Autodesk Inventor part; units mm, degrees
ref_plane "YZ Plane" through (0, 0, 0) normal (1, 0, 0) x (0, 1, 0)
ref_plane "XZ Plane" through (0, 0, 0) normal (0, 1, 0) x (-1, 0, 0)
ref_plane "XY Plane" through (0, 0, 0) normal (0, 0, 1) x (1, 0, 0)
sketch "Sketch1" plane through (0, 0, 0) normal (1, 0, 0) x (0, 1, 0)
  line L0 (1.27, -4.5) -> (-1.27, -4.5)
  line L1 (-1.27, -4.5) -> (-1.27, 4.5)
  line L2 (-1.27, 4.5) -> (1.27, 4.5)
  line L3 (1.27, 4.5) -> (1.27, -4.5)
  line L4 (1.27, -4.5) -> (-1.27, 4.5) construction
  line L5 (-1.27, -4.5) -> (1.27, 4.5) construction
  point P0 (0, 0)
  point P1 (0, 0)
  dimension "d0" = 9
  dimension "d1" = 2.54
sketch "Sketch2" plane through (0, 0, 0) normal (0, 0, 1) x (1, 0, 0)
  arc A0 (-41.75, 0) -> (-41.75, -35.0141) centre (-41.75, -17.507) ccw
  arc A1 (41.75, -35.0141) -> (41.75, 0) centre (41.75, -17.507) ccw
  line L0 (-41.75, 0) -> (41.75, 0)
  line L1 (41.75, -35.0141) -> (-41.75, -35.0141)
  point P0 (0, 0)
  point P1 (0, 0)
  dimension "d2" = 83.5
  dimension "d3" = 17.507
sweep "Sweep1" add profiles "Sketch1" path "Sketch2"
properties part number "55t_Belt" material "Rubber"
Model file for the job. Use its own axes, mm. A direction names the side the tool comes from. Round coordinates to 2 decimals unless told otherwise and drop trailing zeros. Loops run counter-clockwise (first coordinate to the right, second up) from the corner with the lowest first, then second, coordinate; pieces in that order, holes last.
1. Wall check: probe 1 along Y at (x, z) = (-40, -3); probe 2 along X at (y, z) = (-11.5, -2.5); probe 3 along X at (y, z) = (-16.5, 2.25). Give the ranges that are in metal, low to high.
Check values:
probe 1: y = -36.28 to -33.74, -1.27 to 1.27
probe 2: x = -59.54 to -56.83, 56.84 to 59.54
probe 3: x = -60.5 to -57.96, 57.96 to 60.5
2. Tool access for faces 5 (the cylindrical face through (-57.983, -17.864, -0.063)), 6 (the cylindrical face through (-60.522, -17.094, 0.063)): list every direction of +Z, -Z, +X, -X, +Y, -Y with a clear straight run to the whole face (end or side of a thin tool).
Check values:
face 5: +Z, -Z
face 6: +Z, -Z, -X
3. Drop flat-ended pins along their axis: P1, Ø4, axis at y = -32, z = -2.5, coming from the +X side; P2, Ø4, axis at x = 4.5, y = -30, coming from the -Z side; P3, Ø1.5, axis at y = -10.5, z = -0.5, coming from the +X side; P4, Ø3, axis at y = -7.5, z = -3.5, coming from the +X side. Give the stop position or say it passes through.
Check values:
P1: stops at x = 55.77
P2: passes through
P3: stops at x = 59.45
P4: stops at x = 58.49
4. Band-saw the part on A-A, the plane x = 21.5. List the corners of the cut face in (y, z).
Check values:
outline: (-36.28, -4.5) - (-33.74, -4.5) - (-33.74, 4.5) - (-36.28, 4.5) - close; (-1.27, -4.5) - (1.27, -4.5) - (1.27, 4.5) - (-1.27, 4.5) - close
5. Mould opens along X. For faces 1 (the flat face through (-1, -1.27, 0)), 2 (the cylindrical face through (57.983, -17.15, -0.063)), 3 (the cylindrical face through (60.523, -17.92, 0.063)), 4 (the flat face through (-1, 1.27, 0)) say: +X half, -X half, draft (parallel to the pull), parting line (faces both ways), or undercut.
Check values:
face 1: undercut
face 2: undercut
face 3: +X half
face 4: draft
6. Band-saw the part on C-C, the plane y = -23. List the corners of the cut face in (x, z).
Check values:
outline: (-59.71, -4.5) - (-57.03, -4.5) - (-57.03, 4.5) - (-59.71, 4.5) - close; (57.03, -4.5) - (59.71, -4.5) - (59.71, 4.5) - (57.03, 4.5) - close
7. Band-saw the part on B-B, the plane z = -2.5. List the corners of the cut face in (x, y), and give its area (3 significant figures).
Check values:
outline: (-41.75, -36.28) - (41.75, -36.28) arc R18.78 ccw to (41.75, 1.27) - (-41.75, 1.27) arc R18.78 ccw to start; hole (-41.75, -33.74) - (41.75, -33.74) arc R16.24 ccw to (41.75, -1.27) - (-41.75, -1.27) arc R16.24 ccw to start
area: 704 mm2
